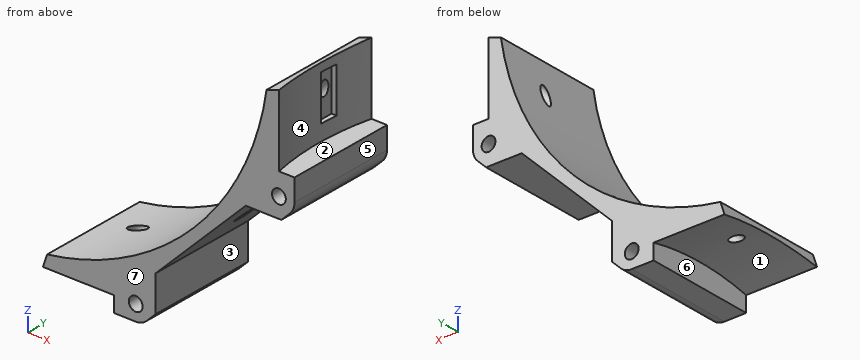
Autodesk Inventor part; units mm, degrees
ref_plane "YZ Plane" through (0, 0, 0) normal (1, 0, 0) x (0, 1, 0)
ref_plane "XZ Plane" through (0, 0, 0) normal (0, 1, 0) x (-1, 0, 0)
ref_plane "XY Plane" through (0, 0, 0) normal (0, 0, 1) x (1, 0, 0)
sketch "Эскиз1" plane through (0, 0, 0) normal (0, 1, 0) x (-1, 0, 0)
  circle A0 centre (-44.87, 82.9015) radius 1.5
  line L0 (-31, 99.2724) -> (-31, 78.7724)
  line L1 (-31, 78.7724) -> (31, 78.7724)
  circle A1 centre (-42.22, 16) radius 1.5
  circle A2 centre (-16, 42.22) radius 1.5
  circle A3 centre (16, 42.22) radius 1.5
  circle A4 centre (31, 72.43) radius 1.5
  circle A5 centre (16, 72.43) radius 1.5
  circle A6 centre (-16, 72.43) radius 1.5
  arc A7 (-31, 99.2724) -> (-99.2724, 31) centre (0, 0) ccw
  circle A8 centre (-74.5664, 57.67) radius 1.5
  circle A9 centre (-82.9015, 44.87) radius 1.5
  circle A10 centre (-72.43, -16) radius 1.5
  circle A11 centre (-72.43, 16) radius 1.5
  line L2 (-78.7724, 31) -> (-78.7724, -31)
  line L3 (-99.2724, 31) -> (-78.7724, 31)
  line L4 (31, 78.7724) -> (31, 99.2724)
  arc A12 (34.57, 98.0863) -> (98.0863, 34.57) centre (109.0212, 109.0212) ccw
  circle A13 centre (72.43, 31) radius 1.5
  line L5 (99.2724, 31) -> (78.7724, 31)
  circle A14 centre (72.43, 16) radius 1.5
  arc A15 (34.57, 98.0863) -> (31, 99.2724) centre (0, 0) ccw
  arc A16 (99.2724, 31) -> (98.0863, 34.57) centre (0, 0) ccw
  arc A17 (98.0863, 34.57) -> (34.57, 98.0863) centre (0, 0) ccw
  circle A18 centre (42.22, 16) radius 1.5
  circle A19 centre (82.9015, -44.87) radius 1.5
  line L6 (78.7724, -31) -> (99.2724, -31)
  arc A20 (31, -99.2724) -> (99.2724, -31) centre (0, 0) ccw
  circle A21 centre (16, -72.43) radius 1.5
  line L7 (31, -78.7724) -> (31, -99.2724)
  circle A22 centre (44.87, -82.9015) radius 1.5
  circle A23 centre (57.67, -74.5664) radius 1.5
  circle A24 centre (-57.67, 74.5664) radius 1.5
  circle A25 centre (-42.22, -16) radius 1.5
  circle A26 centre (42.22, -16) radius 1.5
  circle A27 centre (-72.43, -31) radius 1.5
  line L8 (-73.5391, 73.5391) -> (73.5391, -73.5391) construction
  line L9 (78.7724, 31) -> (78.7724, -31)
  circle A28 centre (72.43, -16) radius 1.5
  circle A29 centre (-16, -42.22) radius 1.5
  circle A30 centre (16, -42.22) radius 1.5
  circle A31 centre (74.5664, -57.67) radius 1.5
  line L10 (-31, -78.7724) -> (31, -78.7724)
  circle A32 centre (-16, -72.43) radius 1.5
  circle A33 centre (-31, -72.43) radius 1.5
  line L11 (-31, -99.2724) -> (-31, -78.7724)
  arc A34 (-34.57, -98.0863) -> (-31, -99.2724) centre (0, 0) ccw
  line L12 (-78.7724, -31) -> (-99.2724, -31)
  arc A35 (-99.2724, -31) -> (-98.0863, -34.57) centre (0, 0) ccw
  arc A36 (-98.0863, -34.57) -> (-34.57, -98.0863) centre (0, 0) ccw
  arc A37 (-34.57, -98.0863) -> (-98.0863, -34.57) centre (-109.0212, -109.0212) ccw
sketch "Эскиз2" plane through (0, 0, 0) normal (0, 1, 0) x (-1, 0, 0)
  arc A0 (34.57, 98.0863) -> (98.0863, 34.57) centre (109.0212, 109.0212) ccw
  arc A1 (99.2724, 31) -> (98.0863, 34.57) centre (0, 0) ccw
  arc A2 (34.57, 98.0863) -> (31, 99.2724) centre (0, 0) ccw
  line L0 (31, 78.7724) -> (31, 99.2724)
  circle A3 centre (31, 72.43) radius 1.5
  circle A4 centre (72.43, 31) radius 1.5
  circle A5 centre (31, 72.43) radius 4.5
  circle A6 centre (72.43, 31) radius 4.5
  line L1 (27.818, 69.248) -> (69.248, 27.818)
  line L2 (26.5, 78.7724) -> (26.5, 72.43)
  line L3 (78.7724, 31) -> (78.7724, -31)
  line L4 (78.7724, 26.5) -> (72.43, 26.5)
  line L5 (99.2724, 31) -> (78.7724, 31)
  line L6 (26.5, 78.7724) -> (31, 78.7724)
  dimension "d0" = 9
  dimension "d1" = 9
extrude "Выдавливание1" add sketch "Эскиз2" along normal blind 32
ref_plane "РабПлоскость1" through (0, 25.3, 0) normal (0, 1, 0) x (1, 0, 0)
sketch "Эскиз3" plane through (0, 25.3, 0) normal (0, 1, 0) x (1, 0, 0)
  circle A0 centre (-72.43, -31) radius 1.5
  circle A1 centre (-31, -72.43) radius 1.5
  point P0 (0, 0)
extrude "Выдавливание2" add sketch "Эскиз3" against normal blind 20.6
sketch "Эскиз4" plane through (-31, 0, 78.7724) normal (0, 0, 1) x (1, 0, 0)
  line L0 (0, 1) -> (0, 32)
  line L1 (0, 32) -> (-3.57, 32)
  line L2 (0, 0) -> (0, 32)
  arc A0 (0, 32) -> (0, 0) centre (72.5929, 16) ccw
  point P0 (31, 0)
extrude "Выдавливание3" cut sketch "Эскиз4" along normal through all
ref_plane "РабПлоскость2" through (-48.533, 0, 48.533) normal (0.7071, 0, 0.7071) x (0, 1, 0)
mirror "Зеркальное отражение1" about plane through (-48.533, 0, 48.533) normal (0.7071, 0, 0.7071) of "Выдавливание3"
ref_plane "РабПлоскость3" through (-98.0863, 32, 34.57) normal (0.7071, 0, -0.7071) x (0.7071, 0, 0.7071)
sketch "Эскиз6" plane through (-98.0863, 32, 34.57) normal (0.7071, 0, -0.7071) x (0.7071, 0, 0.7071)
  line L0 (0, -5.66) -> (89.8256, -5.66)
  line L1 (89.8256, -5.66) -> (89.8256, 35)
  line L2 (89.8256, 35) -> (0, 35)
  line L3 (0, 35) -> (0, -5.66)
  circle A0 centre (45.1056, 17) radius 2
  line L4 (89.8256, 32) -> (89.8256, 0)
  line L5 (89.8256, 32) -> (89.8256, 35)
  point P0 (44.9128, 32)
  dimension "d12" = 3
hole "Отверстие1" at (-66.1918, 15, 66.4645) direction (0.7071, 0, -0.7071) diameter 5.5 end through all
sketch "Эскиз7" plane through (0, 32, 0) normal (0, 1, 0) x (1, 0, 0)
  line L0 (-31, -78.7724) -> (-26.5, -78.7724) construction
  line L1 (-78.7724, -26.5) -> (-78.7724, -31) construction
  line L2 (-31, -78.7724) -> (-78.7724, -31) construction
  arc A0 (-34.57, -98.0863) -> (-98.0863, -34.57) centre (-109.0212, -109.0212) ccw construction
  line L3 (-40.6087, -66.7716) -> (-66.7716, -40.6087)
  line L4 (-66.7716, -40.6087) -> (-66.7716, -30.2944)
  line L5 (-66.7716, -40.6087) -> (-61.6145, -35.4515) construction
  line L6 (152.6297, 152.6297) -> (-152.6297, -152.6297) construction
  line L7 (-61.6145, -35.4515) -> (-66.7716, -30.2944) construction
  line L8 (-27.818, -69.248) -> (-69.248, -27.818) construction
  line L9 (-40.6087, -66.7716) -> (-30.2944, -66.7716)
  line L10 (-40.6087, -66.7716) -> (-35.4515, -61.6145) construction
  line L11 (-35.4515, -61.6145) -> (-30.2944, -66.7716) construction
  line L12 (-30.2944, -66.7716) -> (-66.7716, -30.2944)
  point P0 (0, 0)
  point P1 (-55.8115, -55.8115)
  point P2 (-53.6901, -53.6901)
  dimension "d20" = 3
  dimension "d21" = 37
extrude "Выдавливание4" cut sketch "Эскиз7" against normal through all
ref_plane "РабПлоскость4" through (0, 19.2, 0) normal (0, 1, 0) x (1, 0, 0)
sketch "Эскиз9" plane through (0, 32, 0) normal (0, 1, 0) x (1, 0, 0)
  arc A0 (-98.0863, -34.57) -> (-34.57, -98.0863) centre (0, 0) ccw
  arc A1 (-34.57, -98.0863) -> (-98.0863, -34.57) centre (-109.0212, -109.0212) ccw construction
  line L0 (-73.5391, -73.5391) -> (-55.8115, -55.8115)
  line L1 (-89.442, -36.363) -> (-31, -94.805)
  line L2 (-31, -99.2724) -> (-31, -78.7724) construction
  line L3 (-218.9579, 86.3016) -> (86.3016, -218.9579)
  line L4 (-32.7423, -78.7724) -> (-32.7423, -98.7114)
  line L5 (-25, -115) -> (25, -115) construction
  line L6 (25, -115) -> (25, -87) construction
  line L7 (25, -87) -> (-25, -87) construction
  line L8 (-25, -87) -> (-25, -115) construction
  line L9 (31, -78.7724) -> (-31, -78.7724)
  line L10 (0, -78.7724) -> (0, -128.7724) construction
  line L11 (-37, -86) -> (-32.6866, -81.6866)
  line L12 (-32.6866, -81.6866) -> (-24.2014, -90.1719)
  line L13 (-24.2014, -90.1719) -> (-28.5147, -94.4853)
  line L14 (-28.5147, -94.4853) -> (-37, -86)
  point P0 (-62.9025, -62.9025)
  point P1 (0, -87)
  dimension "d25" = 17.7276
  dimension "d26" = 7.0911
  dimension "d35" = 50
  dimension "d36" = 50
  dimension "d38" = 6.1
  dimension "d39" = 12
sketch "Эскиз10" plane through (0, 19.2, 0) normal (0, 1, 0) x (1, 0, 0)
  line L0 (-34, -83.2724) -> (-34, -96.2724)
  line L1 (-34, -96.2724) -> (-31, -96.2724)
  line L2 (-31, -96.2724) -> (-31, -83.2724)
  line L3 (-31, -83.2724) -> (-34, -83.2724)
  line L4 (-31, -99.2724) -> (-31, -78.7724)
  arc A0 (-34.57, -98.0863) -> (-31, -99.2724) centre (0, 0) ccw
  point P0 (-31, -99.2724)
  dimension "d40" = 3
  dimension "d41" = 13
  dimension "d65" = 3
extrude "Выдавливание6" cut sketch "Эскиз10" along normal mid plane 5.15
sketch "Эскиз11" plane through (-63.5, 13.425, 63.5) normal (0.7071, 0, 0.7071) x (0.7071, 0, -0.7071)
  circle A0 centre (1.6, 5.775) radius 1.5
  line L0 (15.3638, -13.425) -> (15.3638, 18.575)
  line L1 (6.8785, 3.2) -> (6.8785, 8.35)
  line L2 (6.8785, 5.775) -> (3.3286, 5.775)
  point P0 (89.8026, -13.425)
  dimension "d45" = 3
  dimension "d48" = 13.7638
extrude "Выдавливание7" cut sketch "Эскиз11" along normal mid plane 100
sketch "Эскиз12" plane through (0, 32, 0) normal (0, 1, 0) x (1, 0, 0)
  circle A0 centre (-72.43, -31) radius 1.5
  circle A1 centre (-31, -72.43) radius 1.5
  point P0 (0, 0)
hole "Отверстие2" at (-72.43, 32, 31) at (-31, 32, 72.43) direction (0, -1, 0) diameter 4 depth 4.7
hole "Отверстие3" at (-31, 0, 72.43) at (-72.43, 0, 31) direction (0, 1, 0) diameter 4 depth 4.7
equation "\"d1\" = d0"
properties part number "kicker_cetch"
Read the model definition and answer for the solid it produces. Units are mm, in the model's axes. Face numbers are marked on the shaded views. A direction names the side the tool comes from. Coordinates: 2 decimals unless noted, no trailing zeros. Loops run counter-clockwise (first coordinate to the right, second up) from the corner with the lowest first, then second, coordinate; pieces in that order, holes last.
(1) Flat-ended cylindrical pins translate along their axes: pin 1 Ø1.9 at (y, z) = (10, 31) entering from -X; pin 2 Ø3.5 at (x, z) = (-31, 72.43) entering from +Y; pin 3 Ø2 at (x, z) = (-31, 72) entering from +Y. Find the tip coordinate at first contact, or state that the pin passes through.
Solution:
pin 1: stops at x = -78.77
pin 2: stops at y = 27.3
pin 3: stops at y = 25.3
(2) The part is cut by section C-C (x = -39). Determine the outline of the cut face in (y, z), and give its area (3 significant figures).
Solution:
outline: (0, 66.77) - (32, 66.77) - (32, 81.46) - (0, 81.46) - close
area: 470 mm2
(3) The mould has two halves that part along Y. Classify the marked faces 4, 5, 6 and 7: released by +Y, released by -Y, zero draft, split by the parting line, or undercut.
Solution:
face 4: undercut
face 5: zero draft
face 6: undercut
face 7: released by -Y
(4) Consider line 1 along X through (y, z) = (26.75, 31); line 2 along Z through (x, y) = (-31, 26); line 3 along Z through (x, y) = (-72, 26). Determine where each line is inside the solid, lowest interval first.
Solution:
line 1: x = -78.77 to -73.93, -70.93 to -66.77
line 2: z = 66.77 to 70.93, 73.93 to 78.77
line 3: z = 26.52 to 29.56, 32.44 to 43.51
(5) The part is cut by section B-B (z = 68). Determine the outline of the cut face in (x, y), and give its area (3 significant figures).
Solution:
outline: (-45.94, 0) - (-29.07, 0) - (-29.07, 32) - (-45.94, 32) - close
area: 540 mm2
(6) The part is cut by section A-A (y = 8.5). Determine the outline of the cut face in (x, z).
Solution:
outline: (-98.84, 32.36) - (-78.77, 32.36) - (-78.77, 26.5) - (-72.43, 26.5) arc R4.5 ccw to (-69.25, 27.82) - (-66.77, 30.29) - (-66.77, 40.61) - (-40.61, 66.77) - (-30.29, 66.77) - (-27.82, 69.25) arc R4.5 ccw to (-26.5, 72.43) - (-26.5, 78.77) - (-32.36, 78.77) - (-32.36, 98.84) arc R104.03 ccw to (-34.57, 98.09) arc R75.25 cw to (-98.09, 34.57) arc R103.97 ccw to start
(7) A tool of negligible diameter and unlimited length cuts with its end or side. For the marked faces 1, 2 and 3, from which of +Z, -Z, +X, -X, +Y, -Y can it reach the whole face along a straight path? Write none if from no direction.
Solution:
face 1: -Z, -X
face 2: +Z, +X
face 3: -Z, +X, +Y, -Y
